```python
from build123d import *
from OCP.BRepFilletAPI import BRepFilletAPI_MakeChamfer

# Parameters (mm, degrees)
SKETCH1_W            = 390.7
SKETCH1_H            = 132.7
MAINBODY_DEPTH       = 18.5
SKETCH2_W            = 390.7
SKETCH2_H            = 132.7
SKETCH2_W_2          = 386.7
SKETCH2_H_2          = 128.7
ALIGMENTLIP_DEPTH    = 2
TYPINGANGLE_DEPTH    = 414.035143783
SKETCH4_W            = 372
SKETCH4_H            = 120
PCBCUTOUT_DEPTH      = 3
M3_CLEARANCE_HOLE1_D = 3.4
CUT_EXTRUDE2_START   = -1
SKETCH11_R           = 3.25
CUT_EXTRUDE2_DEPTH   = 412.911649145
SKETCH12_W           = 15
SKETCH12_H           = 3.5
CUT_EXTRUDE3_DEPTH   = 3
FILLET1_R            = 2.5
SKETCH13_W           = 15
SKETCH13_H           = 20
CUT_EXTRUDE4_DEPTH   = 2
FILLET2_R            = 4
CHAMFER1_SIZE        = 0.5
CHAMFER1_SIZE2       = 0.561801899
CHAMFER2_SIZE        = 0.5
SKETCH17_R           = 1
SKETCH17_W           = 2
SKETCH17_H           = 2
CUT_EXTRUDE5_DEPTH   = 1


with BuildPart() as part:
    # Sketch1 → MainBody (new body)
    with BuildSketch(Plane(origin=(0, 0, 0), x_dir=(1, 0, 0), z_dir=(0, 1, 0))):
        with Locations((195.35, 66.35)):
            Rectangle(SKETCH1_W, SKETCH1_H)
    extrude(amount=MAINBODY_DEPTH)

    # Sketch2 → AligmentLip (cut)
    with BuildSketch(Plane(origin=(0, 18.5, 0), x_dir=(1, 0, 0), z_dir=(0, 1, 0))):
        with Locations((195.35, 66.35)):
            Rectangle(SKETCH2_W, SKETCH2_H)
        with Locations((195.35, 66.35)):
            Rectangle(SKETCH2_W_2, SKETCH2_H_2, mode=Mode.SUBTRACT)
    extrude(amount=-ALIGMENTLIP_DEPTH, mode=Mode.SUBTRACT)

    # Sketch3 → TypingAngle (cut, through all)
    with BuildSketch(Plane.ZY):
        Polygon((-116.028888387, 0), (-132.7, 13.5), (-132.7, 0), align=None)
        Polygon((0, 12.195127583), (-116.028888387, 0), (0, 0), align=None)
    extrude(amount=-TYPINGANGLE_DEPTH, mode=Mode.SUBTRACT)

    # Sketch4 → PCBCutout (cut)
    with BuildSketch(Plane(origin=(0, 18.5, 0), x_dir=(1, 0, 0), z_dir=(0, 1, 0))):
        with Locations((195.35, 66.35)):
            Rectangle(SKETCH4_W, SKETCH4_H)
    extrude(amount=-PCBCUTOUT_DEPTH, mode=Mode.SUBTRACT)

    # M3 Clearance Hole1 (through all)
    with Locations(Plane(origin=(110, 18.5, -128.3), x_dir=(0, 0, 1), z_dir=(0, 1, 0))):
        with Locations((0, 0), (16.95, -104.3), (61.95, -104.3), (106.95, -104.3), (123.9, 0), (0, 170.7), (123.9, 170.7), (106.95, 275), (61.95, 275), (16.95, 275)):
            Hole(M3_CLEARANCE_HOLE1_D / 2)

    # Sketch11 → Cut-Extrude2 (cut, through all)
    with BuildSketch(Plane(origin=(0, 15.5, 0), x_dir=(1, 0, 0), z_dir=(0, 1, 0)).offset(CUT_EXTRUDE2_START)):
        with Locations(Location((110, 128.3, 0), (0, 0, 270))):
            Circle(SKETCH11_R)
        with Locations(Location((5.7, 111.35, 0), (0, 0, 270))):
            Circle(SKETCH11_R)
        with Locations(Location((5.7, 66.35, 0), (0, 0, 270))):
            Circle(SKETCH11_R)
        with Locations(Location((5.7, 21.35, 0), (0, 0, 270))):
            Circle(SKETCH11_R)
        with Locations(Location((110, 4.4, 0), (0, 0, 270))):
            Circle(SKETCH11_R)
        with Locations(Location((280.7, 4.4, 0), (0, 0, 270))):
            Circle(SKETCH11_R)
        with Locations(Location((385, 21.35, 0), (0, 0, 270))):
            Circle(SKETCH11_R)
        with Locations(Location((385, 66.35, 0), (0, 0, 270))):
            Circle(SKETCH11_R)
        with Locations(Location((385, 111.35, 0), (0, 0, 270))):
            Circle(SKETCH11_R)
        with Locations(Location((280.7, 128.3, 0), (0, 0, 90))):
            Circle(SKETCH11_R)
    extrude(amount=-CUT_EXTRUDE2_DEPTH, mode=Mode.SUBTRACT)

    # Sketch12 → Cut-Extrude3 (cut)
    with BuildSketch(Plane(origin=(0, 18.5, 0), x_dir=(1, 0, 0), z_dir=(0, 1, 0))):
        with Locations((35.9, 128.1)):
            Rectangle(SKETCH12_W, SKETCH12_H)
    extrude(amount=-CUT_EXTRUDE3_DEPTH, mode=Mode.SUBTRACT)

    # Fillet1
    fillet1_edges = [part.edges().sort_by_distance(p)[0] for p in [
        (28.4, 17, -129.85),
        (43.4, 17, -129.85),
    ]]
    fillet(fillet1_edges, radius=FILLET1_R)

    # Sketch13 → Cut-Extrude4 (cut)
    with BuildSketch(Plane(origin=(0, 15.5, 0), x_dir=(1, 0, 0), z_dir=(0, 1, 0))):
        with Locations((16.85, 66.35)):
            Rectangle(SKETCH13_W, SKETCH13_H)
    extrude(amount=-CUT_EXTRUDE4_DEPTH, mode=Mode.SUBTRACT)

    # Fillet2
    fillet2_edges = [part.edges().sort_by_distance(p)[0] for p in [
        (388.7, 17.5, -130.7),
        (2, 17.5, -130.7),
        (2, 17.5, -2),
        (388.7, 17.5, -2),
        (9.35, 14.5, -56.35),
        (9.35, 14.5, -76.35),
        (24.35, 14.5, -76.35),
        (24.35, 14.5, -56.35),
        (9.35, 17, -6.35),
        (9.35, 17, -126.35),
        (381.35, 17, -126.35),
        (381.35, 17, -6.35),
    ]]
    fillet(fillet2_edges, radius=FILLET2_R)

    # Chamfer1: one chamfer whose edges measure the first distance from different faces: ONE call of the kernel's chamfer builder (chamfer() names one face for all edges)
    chamfer1_edges_1 = [part.edges().sort_by_distance(p)[0] for p in [
        (0, 15, -132.7),
        (390.7, 15, -132.7),
        (390.7, 14.347563791, 0),
        (0, 14.347563791, 0),
        (195.35, 16.5, -132.7),
        (390.7, 16.5, -66.35),
        (195.35, 16.5, 0),
        (0, 16.5, -66.35),
        (0, 6.75, -124.364444193),
        (390.7, 6.75, -124.364444193),
        (0, 6.097563791, -58.014444193),
        (390.7, 6.097563791, -58.014444193),
    ]]
    chamfer1_edges_2 = [part.edges().sort_by_distance(p)[0] for p in [
        (195.35, 12.195127583, 0),
    ]]
    chamfer1_side_2 = [part.faces().sort_by_distance(p)[0] for p in [
        (195.35, 14.347563791, 0),
    ]]
    chamfer1 = BRepFilletAPI_MakeChamfer(part.part.solid().wrapped)
    for e in chamfer1_edges_1:
        chamfer1.Add(CHAMFER1_SIZE, e.wrapped)
    for e in chamfer1_edges_2:
        chamfer1.Add(CHAMFER1_SIZE, CHAMFER1_SIZE2, e.wrapped, chamfer1_side_2[0].wrapped)  # the first distance lies on this face
    add(Compound.cast(chamfer1.Shape()), mode=Mode.REPLACE)

    # Chamfer2
    chamfer2_edges = [part.edges().sort_by_distance(p)[0] for p in [
        (388.7, 18.5, -66.35),
        (195.35, 18.5, -130.7),
        (2, 18.5, -66.35),
        (195.35, 18.5, -2),
        (3.171572875, 18.5, -129.528427125),
        (3.171572875, 18.5, -3.171572875),
        (387.528427125, 18.5, -3.171572875),
        (387.528427125, 18.5, -129.528427125),
    ]]
    chamfer(chamfer2_edges, length=CHAMFER2_SIZE)

    # Sketch17 → Cut-Extrude5 (cut)
    with BuildSketch(Plane(origin=(0, 12.061881184, -1.267754798), x_dir=(1, 0, 0), z_dir=(0, -0.9945218953682734, 0.10452846326765429))):
        with Locations((205.1, -52.225262054)):
            Circle(SKETCH17_R)
        with BuildLine():
            ThreePointArc((204.1, -52.225262054), (205.1, -51.225262054), (206.1, -52.225262054))
            Line((206.1, -52.225262054), (206.1, -49.725262054))
            ThreePointArc((206.1, -49.725262054), (205.1, -50.725262054), (204.1, -49.725262054))
            Line((204.1, -49.725262054), (204.1, -52.225262054))
        make_face()
        with Locations((205.1, -49.725262054)):
            Circle(SKETCH17_R)
        with Locations((201.6, -49.725262054)):
            Circle(SKETCH17_R)
        with BuildLine():
            ThreePointArc((200.6, -60.225262054), (201.6, -59.225262054), (202.6, -60.225262054))
            Line((202.6, -60.225262054), (202.6, -49.725262054))
            ThreePointArc((202.6, -49.725262054), (201.6, -50.725262054), (200.6, -49.725262054))
            Line((200.6, -49.725262054), (200.6, -60.225262054))
        make_face()
        with Locations((201.6, -60.225262054)):
            Circle(SKETCH17_R)
        with Locations((197.1, -53.725262054)):
            Circle(SKETCH17_R)
        with BuildLine():
            Line((196.1, -62.725262054), (198.1, -62.725262054))
            Line((198.1, -62.725262054), (198.1, -53.725262054))
            ThreePointArc((198.1, -53.725262054), (197.1, -54.725262054), (196.1, -53.725262054))
            Line((196.1, -53.725262054), (196.1, -62.725262054))
        make_face()
        with Locations((197.1, -63.725262054)):
            Rectangle(SKETCH17_W, SKETCH17_H)
        with BuildLine():
            ThreePointArc((196.1, -67.725262054), (197.1, -66.725262054), (198.1, -67.725262054))
            Line((198.1, -67.725262054), (198.1, -64.725262054))
            Line((198.1, -64.725262054), (196.1, -64.725262054))
            Line((196.1, -64.725262054), (196.1, -67.725262054))
        make_face()
        with Locations((197.1, -67.725262054)):
            Circle(SKETCH17_R)
        with BuildLine():
            Line((194.1, -64.725262054), (196.1, -64.725262054))
            Line((196.1, -64.725262054), (196.1, -62.725262054))
            Line((196.1, -62.725262054), (194.1, -62.725262054))
            ThreePointArc((194.1, -62.725262054), (194.807106781, -63.018155273), (195.1, -63.725262054))
            ThreePointArc((195.1, -63.725262054), (194.807106781, -64.432368836), (194.1, -64.725262054))
        make_face()
        with Locations((194.1, -63.725262054)):
            Circle(SKETCH17_R)
        with Locations(Location((201.6, -63.725262054, 0), (0, 0, 270))):
            Circle(SKETCH17_R)
        with Locations((192.6, -60.225262054)):
            Circle(SKETCH17_R)
        with BuildLine():
            ThreePointArc((191.6, -60.225262054), (192.6, -59.225262054), (193.6, -60.225262054))
            Line((193.6, -60.225262054), (193.6, -54.225262054))
            ThreePointArc((193.6, -54.225262054), (192.6, -55.225262054), (191.6, -54.225262054))
            Line((191.6, -54.225262054), (191.6, -60.225262054))
        make_face()
        with Locations((192.6, -54.225262054)):
            Circle(SKETCH17_R)
        with BuildLine():
            ThreePointArc((188.1, -60.225262054), (189.1, -59.225262054), (190.1, -60.225262054))
            Line((190.1, -60.225262054), (190.1, -54.225262054))
            ThreePointArc((190.1, -54.225262054), (189.1, -55.225262054), (188.1, -54.225262054))
            Line((188.1, -54.225262054), (188.1, -60.225262054))
        make_face()
        with Locations((189.1, -60.225262054)):
            Circle(SKETCH17_R)
        with Locations((189.1, -54.225262054)):
            Circle(SKETCH17_R)
        with Locations((185.6, -54.225262054)):
            Circle(SKETCH17_R)
        with BuildLine():
            ThreePointArc((184.6, -60.225262054), (185.6, -59.225262054), (186.6, -60.225262054))
            Line((186.6, -60.225262054), (186.6, -54.225262054))
            ThreePointArc((186.6, -54.225262054), (185.6, -55.225262054), (184.6, -54.225262054))
            Line((184.6, -54.225262054), (184.6, -60.225262054))
        make_face()
        with Locations((185.6, -60.225262054)):
            Circle(SKETCH17_R)
    extrude(amount=-CUT_EXTRUDE5_DEPTH, mode=Mode.SUBTRACT)


solid = part.part
```
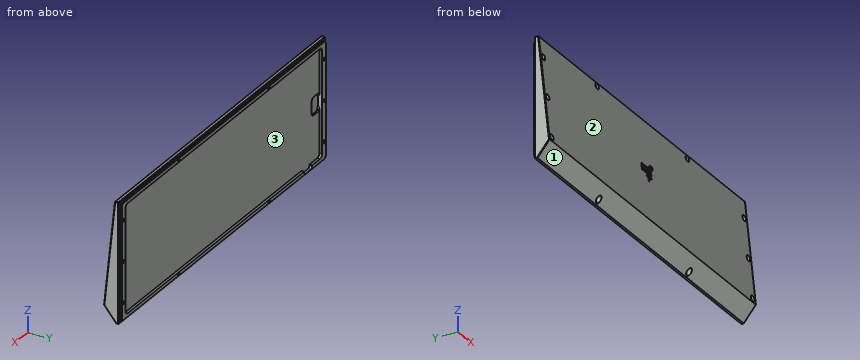
Geometry check sheet. Reference: the model listing, model coordinates, mm. Face numbers are marked on the shaded views. Round coordinates to 2 decimals unless told otherwise and drop trailing zeros. Loops run counter-clockwise (first coordinate to the right, second up) from the corner with the lowest first, then second, coordinate; pieces in that order, holes last. Notation, with made-up numbers: (-34, 16) -> (23, 16) arc R27 cw to (23, 35) -> close; hole circle Ø2 at (-11.5, 36.5). An arc over 180 degrees is marked (long way). Use a Markdown table: item, result.
(1) Scan lines: probe 1 along Z at (x, y) = (110, 16.65); probe 2 along X at (y, z) = (17.05, -111.35); probe 3 along Z at (x, y) = (385, 16.55). Record each from-to range of solid material in increasing order.
Calculated:
| item | result |
|---|---|
| probe 1 | -130.7 to -130, -126.6 to -126.35, -6.35 to -6.1, -2.7 to -2 |
| probe 2 | 2 to 4, 7.4 to 9.35, 381.35 to 383.3, 386.7 to 388.7 |
| probe 3 | -130.69 to -113.05, -109.65 to -68.05, -64.65 to -23.05, -19.65 to -2.01 |
(2) Sectioned sample at B-B (z = -29.5). Enter the section's corners in (x, y).
Calculated:
| item | result |
|---|---|
| outline | (0, 9.6) -> (0.5, 9.09) -> (390.2, 9.09) -> (390.7, 9.6) -> (390.7, 16) -> (390.2, 16.5) -> (388.7, 16.5) -> (388.7, 18) -> (388.2, 18.5) -> (381.35, 18.5) -> (381.35, 15.5) -> (9.35, 15.5) -> (9.35, 18.5) -> (2.5, 18.5) -> (2, 18) -> (2, 16.5) -> (0.5, 16.5) -> (0, 16) -> close |
(3) Mould release check, pull along Z, two halves, no side actions. Record for the marked faces 1, 2 and 3: released by +Z, released by -Z, zero draft, split by the parting line, or undercut.
Calculated:
| item | result |
|---|---|
| face 1 | released by -Z |
| face 2 | released by +Z |
| face 3 | undercut |
(4) Go/stop test with flat-tipped pins: P1, Ø10, axis at x = 295.5, z = -69.5, coming from the -Y side; P2, Ø4, axis at x = 190.5, z = -25.5, coming from the -Y side; P3, Ø3, axis at x = 281.5, z = -4, coming from the -Y side. Record where each tip stops, or that it passes through.
Calculated:
| item | result |
|---|---|
| P1 | y = 4.36 |
| P2 | y = 9.3 |
| P3 | y = 14.5 |
(5) Sectioned sample at A-A (x = 263). Enter the section's corners in (y, z).
Calculated:
| item | result |
|---|---|
| outline | (0, -116.03) -> (13.5, -132.7) -> (16, -132.7) -> (16.5, -132.2) -> (16.5, -130.7) -> (18, -130.7) -> (18.5, -130.2) -> (18.5, -126.35) -> (15.5, -126.35) -> (15.5, -6.35) -> (18.5, -6.35) -> (18.5, -2.5) -> (18, -2) -> (16.5, -2) -> (16.5, -0.5) -> (16, 0) -> (12.7, 0) -> (12.14, -0.56) -> close |
